```python
from build123d import *

# Parameters (mm, degrees)
SKETCH022_W     = 70
SKETCH022_H     = 65
PAD002_DEPTH    = 1870
POCKET024_DEPTH = 15
POCKET026_DEPTH = 15
SKETCH023_W     = 10
SKETCH023_H     = 30
POCKET019_DEPTH = 70.001
SKETCH024_W     = 20
SKETCH024_H     = 25
POCKET020_DEPTH = 3814.8775
SKETCH025_W     = 50
SKETCH025_H     = 15
POCKET021_DEPTH = 3814.8775
SKETCH029_W     = 10
SKETCH029_H     = 32
POCKET025_DEPTH = 1870.001
SKETCH031_W     = 10
SKETCH031_H     = 32.5
POCKET027_DEPTH = 1870.001


with BuildPart() as part:
    # Sketch022 (on DatumPlane) → Pad002 (new body)
    with BuildSketch(Plane.XY.offset(935)):
        Rectangle(SKETCH022_W, SKETCH022_H)
    extrude(amount=-PAD002_DEPTH)

    # Sketch028 (on DatumPlane) → Pocket024 (cut)
    with BuildSketch(Plane(origin=(0, 0.5, 0), x_dir=(-1, 0, 0), z_dir=(0, 1, 0))):
        Polygon((-35, 890), (15, 890), (15, 935), (35, 935), (35, 820), (-35, 820), align=None)
    extrude(amount=-POCKET024_DEPTH, mode=Mode.SUBTRACT)

    # Sketch030 (on DatumPlane) → Pocket026 (cut)
    with BuildSketch(Plane(origin=(0, 0.5, 0), x_dir=(-1, 0, 0), z_dir=(0, 1, 0))):
        Polygon((35, -770), (-35, -770), (-35, -870), (15, -870), (15, -935), (35, -935), align=None)
    extrude(amount=-POCKET026_DEPTH, mode=Mode.SUBTRACT)

    # Sketch023 (on DatumPlane) → Pocket019 (cut, through all)
    with BuildSketch(Plane.YZ.offset(35)):
        with Locations((-4.5, -305)):
            Rectangle(SKETCH023_W, SKETCH023_H)
        with Locations((-4.5, 175)):
            Rectangle(SKETCH023_W, SKETCH023_H)
        with Locations((-4.5, 655)):
            Rectangle(SKETCH023_W, SKETCH023_H)
    extrude(amount=-POCKET019_DEPTH, mode=Mode.SUBTRACT)

    # Sketch024 (on DatumPlane) → Pocket020 (cut, through all)
    with BuildSketch(Plane.YZ.offset(35)):
        with Locations((22.5, 922.5)):
            Rectangle(SKETCH024_W, SKETCH024_H)
    pocket020 = extrude(amount=-POCKET020_DEPTH, mode=Mode.SUBTRACT)

    # Sketch025 (on DatumPlane) → Pocket021 (cut, through all)
    with BuildSketch(Plane.YZ.offset(35)):
        with Locations((7.5, 927.5)):
            Rectangle(SKETCH025_W, SKETCH025_H)
    pocket021 = extrude(amount=-POCKET021_DEPTH, mode=Mode.SUBTRACT)

    # Mirrored003: Pocket020, Pocket021 across XY
    add(pocket020.mirror(Plane.XY), mode=Mode.SUBTRACT)
    add(pocket021.mirror(Plane.XY), mode=Mode.SUBTRACT)

    # Sketch029 (on DatumPlane) → Pocket025 (cut, through all)
    with BuildSketch(Plane.XY.offset(935)):
        with Locations((-30, 16.5)):
            Rectangle(SKETCH029_W, SKETCH029_H)
    extrude(amount=-POCKET025_DEPTH, mode=Mode.SUBTRACT)

    # Sketch031 (on DatumPlane) → Pocket027 (cut, through all)
    with BuildSketch(Plane.XY.offset(935)):
        with Locations((30, -16.25)):
            Rectangle(SKETCH031_W, SKETCH031_H)
    extrude(amount=-POCKET027_DEPTH, mode=Mode.SUBTRACT)


solid = part.part
```
Check sheet for the modelled part. Datum: model origin and axes. Units: mm. A direction names the side the tool comes from. Coordinates: 2 decimals unless noted, no trailing zeros. Order: outer loops, then holes, each group sorted by start corner. A loop starts at its lowest first (then second) coordinate and runs counter-clockwise, first axis right, second up. Notation, with made-up numbers: (-36.5, 12.5) -> (3.5, 12.5) arc R14 cw to (3.5, 25.5) -> close; hole circle Ø2 at (-33.75, -17.5). An arc over 180 degrees is marked (long way). Write item = value, one per line. Start each with the question number.
1) Material ranges on L1, parallel to Z at x = -6, y = -9; L2, parallel to Y at x = -24, z = -798.5; L3, parallel to X at y = -18.5, z = -214, recorded low to high.
2) Mould release check, pull along Z, two halves, no side actions. Record for faces 6 (the flat face through (35, 16, 13)), 7 (the flat face through (8, -3, -920)), 8 (the flat face through (5, 0.5, 860)): +Z half, -Z half, draft (parallel to the pull), parting line (faces both ways), or undercut.
3) Cross-section at A-A (z = 350.5). Enter the section's corners in (x, y).
4) Go/stop test with flat-tipped pins: P1, Ø2, axis at y = 23, z = 364.5, coming from the -X side; P2, Ø1, axis at x = 25.5, y = 23, coming from the -Z side; P3, Ø2, axis at y = -17, z = 173, coming from the +X side. Record where each tip stops, or that it passes through.
5) Access from +Z, -Z, +X, -X, +Y, -Y to the whole of each face (thin tool, end or side, straight path). Record for faces 1 (the flat face through (-5, -14.5, -827)), 2 (the flat face through (8, -3, 920)), 3 (the flat face through (-25, 16, 13)), 4 (the flat face through (-5, -9.5, 175)), 5 (the flat face through (25, -16, 13)).
Ans:
q1.L1 = -920 to -870, -770 to -320, -290 to 160, 190 to 640, 670 to 820, 890 to 920
q1.L2 = -32.5 to -14.5, 0.5 to 32.5
q1.L3 = -35 to 25
q2.face_6 = draft
q2.face_7 = -Z half
q2.face_8 = undercut
q3.outline = (-35, -32.5) -> (25, -32.5) -> (25, 0) -> (35, 0) -> (35, 32.5) -> (-25, 32.5) -> (-25, 0.5) -> (-35, 0.5) -> close
q4.P1 = -25
q4.P2 = -910
q4.P3 = 25
q5.face_1 = -X
q5.face_2 = +Z, +X, -X, +Y
q5.face_3 = +Z, -Z, -X, +Y
q5.face_4 = +X, -X
q5.face_5 = +Z, -Z, +X, -Y
